Model file for the job. Use its own axes, mm. A direction names the side the tool comes from. Coordinates: 2 decimals unless noted, no trailing zeros. Order: outer loops, then holes, each group sorted by start corner. A loop starts at its lowest first (then second) coordinate and runs counter-clockwise, first axis right, second up.
from build123d import *
from build123d.topology import SkipClean

# Parameters (mm, degrees)
SKETCH1_R               = 38.1
BOSS_EXTRUDE1_DEPTH     = 76.2
SHELL2_T                = 3.175
SKETCH2_W               = 3
SKETCH2_H               = 82.55
SKETCH2_W_2             = 82.55
SKETCH2_H_2             = 3
BOSS_EXTRUDE2_DEPTH     = 4
CUT_EXTRUDE1_DEPTH      = 99.527366122
CUT_EXTRUDE1_DEPTH_BACK = 99.527366122
SKETCH3_R               = 61.906276858
SKETCH3_R_2             = 41.275
SKETCH4_R               = 20.64
CUT_EXTRUDE2_DEPTH      = 4


with BuildPart() as part:
    # Sketch1 → Boss-Extrude1 (new body)
    with BuildSketch(Plane(origin=(0, 0, 0), x_dir=(1, 0, 0), z_dir=(0, 1, 0))):
        with Locations(Location((0, 0, 0), (0, 0, 90))):
            Circle(SKETCH1_R)
    extrude(amount=BOSS_EXTRUDE1_DEPTH)

    # Shell2
    shell2_openings = [part.faces().sort_by_distance(p)[0] for p in [
        (0, 76.2, 0),
    ]]
    offset(amount=SHELL2_T, openings=shell2_openings, kind=Kind.INTERSECTION)

    # Sketch2 → Boss-Extrude2 (add)
    with BuildSketch(Plane(origin=(0, -3.175, 0), x_dir=(-1, 0, 0), z_dir=(0, -1, 0))):
        Rectangle(SKETCH2_W, SKETCH2_H)
        Polygon((-23.047310797, -34.273854321), (25.47436178, 32.510498564), (23.047310797, 34.273854321), (-25.47436178, -32.510498564), align=None)
        Polygon((-38.791332219, -14.181261217), (39.718383202, 11.328091668), (38.791332219, 14.181261217), (-39.718383202, -11.328091668), align=None)
        Polygon((-39.718383202, 11.328091668), (38.791332219, -14.181261217), (39.718383202, -11.328091668), (-38.791332219, 14.181261217), align=None)
        Polygon((-25.47436178, 32.510498564), (23.047310797, -34.273854321), (25.47436178, -32.510498564), (-23.047310797, 34.273854321), align=None)
        Polygon((-14.181261217, 38.791332219), (11.328091668, -39.718383202), (14.181261217, -38.791332219), (-11.328091668, 39.718383202), align=None)
        Polygon((11.328091668, 39.718383202), (-14.181261217, -38.791332219), (-11.328091668, -39.718383202), (14.181261217, 38.791332219), align=None)
        Polygon((32.510498564, 25.47436178), (-34.273854321, -23.047310797), (-32.510498564, -25.47436178), (34.273854321, 23.047310797), align=None)
        Rectangle(SKETCH2_W_2, SKETCH2_H_2)
        Polygon((-34.273854321, 23.047310797), (32.510498564, -25.47436178), (34.273854321, -23.047310797), (-32.510498564, 25.47436178), align=None)
    extrude(amount=BOSS_EXTRUDE2_DEPTH)

    # Sketch3 → Cut-Extrude1 (cut, two sides: drawn at the far end of the back side and taken through both)
    with SkipClean():  # the faces are left unmerged after this step: merging them gives an invalid solid
        with BuildSketch(Plane.XZ.offset(3.175).offset(-CUT_EXTRUDE1_DEPTH_BACK)):
            Circle(SKETCH3_R)
            with Locations(Location((0, 0, 0), (0, 0, 272.082679548))):
                Circle(SKETCH3_R_2, mode=Mode.SUBTRACT)
        extrude(amount=CUT_EXTRUDE1_DEPTH + CUT_EXTRUDE1_DEPTH_BACK, mode=Mode.SUBTRACT)

    # Sketch4 → Cut-Extrude2 (cut)
    with SkipClean():  # the faces are left unmerged after this step: merging them gives an invalid solid
        with BuildSketch(Plane.XZ.offset(7.175)):
            Circle(SKETCH4_R)
        extrude(amount=-CUT_EXTRUDE2_DEPTH, mode=Mode.SUBTRACT)


solid = part.part
Q1. Drop flat-ended pins along their axis: P1, Ø2.5, axis at x = -13.5, z = 3, coming from the -Y side (3 decimals); P2, Ø3, axis at x = -5.5, z = 10.5, coming from the +Y side; P3, Ø1.2, axis at x = 36, y = -6, coming from the -Z side. Give the stop position or say it passes through.
Established:
P1: stops at y = -3.175
P2: stops at y = 0
P3: stops at z = -13.47
Q2. Cut at B-B, the plane z = -27. List the corners of the cut face in (x, y) (3 decimals).
Established:
outline: (-31.219, -3.175) - (-21.471, -3.175) - (-21.471, -7.175) - (-17.763, -7.175) - (-17.763, -3.175) - (-10.35, -3.175) - (-10.35, -7.175) - (-7.196, -7.175) - (-7.196, -3.175) - (-1.5, -3.175) - (-1.5, -7.175) - (1.5, -7.175) - (1.5, -3.175) - (7.196, -3.175) - (7.196, -7.175) - (10.35, -7.175) - (10.35, -3.175) - (17.763, -3.175) - (17.763, -7.175) - (21.471, -7.175) - (21.471, -3.175) - (31.219, -3.175) - (31.219, 76.2) - (26.881, 76.2) - (26.881, 0) - (-26.881, 0) - (-26.881, 76.2) - (-31.219, 76.2) - close
Q3. Cut at A-A, the plane y = 54. List the corners of the cut face in (x, z) (3 decimals).
Established:
outline: circle Ø82.55 at (0, 0); hole circle Ø76.2 at (0, 0)
Q4. Cut at C-C, the plane z = 29. List the corners of the cut face in (x, y) (3 decimals).
Established:
outline: (-29.37, -3.175) - (-22.924, -3.175) - (-22.924, -7.175) - (-19.216, -7.175) - (-19.216, -3.175) - (-11, -3.175) - (-11, -7.175) - (-7.845, -7.175) - (-7.845, -3.175) - (-1.5, -3.175) - (-1.5, -7.175) - (1.5, -7.175) - (1.5, -3.175) - (7.845, -3.175) - (7.845, -7.175) - (11, -7.175) - (11, -3.175) - (19.216, -3.175) - (19.216, -7.175) - (22.924, -7.175) - (22.924, -3.175) - (29.37, -3.175) - (29.37, 76.2) - (24.711, 76.2) - (24.711, 0) - (-24.711, 0) - (-24.711, 76.2) - (-29.37, 76.2) - close
Q5. Mould opens along Z. For faces 4 (the face through (25.777, -5.147, 16.874)), 5 (the face through (1.5, -5, -31)) say: pulls with the +Z half, pulls with the -Z half, needs draft (parallel to the pull), parting line crosses it, or undercut.
Established:
face 4: undercut
face 5: needs draft
Q6. Which spindle directions (+Z, -Z, +X, -X, +Y, -Y) get a long thin tool onto all of the face, cutting with end or side? Do faces 1 (the face through (31, -5, -1.5)), 2 (the face through (-12.115, -5.203, 16.71)), 3 (the face through (-29.729, -5.147, -8.082)). Say none if no direction does.
Established:
face 1: +X, -X, -Y
face 2: -Y
face 3: -X, -Y
Q7. Probe line 1 (X direction, y = 58, z = 0) (3 decimals); line 2 (Y direction, x = 10, z = -5.5) (3 decimals); line 3 (Y direction, x = -7, z = -25) (3 decimals). List the from-to ranges inside material, lowest first.
Established:
line 1: x = -41.275 to -38.1, 38.1 to 41.275
line 2: y = -3.175 to 0
line 3: y = -7.175 to 0
